Autodesk Inventor part; units mm, degrees
ref_plane "YZ Plane" through (0, 0, 0) normal (1, 0, 0) x (0, 1, 0)
ref_plane "XZ Plane" through (0, 0, 0) normal (0, 1, 0) x (-1, 0, 0)
ref_plane "XY Plane" through (0, 0, 0) normal (0, 0, 1) x (1, 0, 0)
sketch "Sketch1" plane through (0, 0, 0) normal (0, 0, 1) x (1, 0, 0)
  line L0 (0, 0) -> (-228.6, 0)
  line L1 (-228.6, 0) -> (-228.6, 1.5875)
  line L2 (-228.6, 1.5875) -> (-95.25, 25.4)
  line L3 (-95.25, 25.4) -> (0, 25.4)
  line L4 (0, 25.4) -> (0, 0)
  dimension "d0" = 25.4
  dimension "d1" = 228.6
  dimension "d2" = 1.5875
  dimension "d3" = 95.25
extrude "Extrusion1" add sketch "Sketch1" along normal blind 25.4
shell "Shell1" thickness 1.5875 removed faces 2 at (-184.15, 9.525, 8.4667) at (0, 16.9333, 8.4667)
sketch "Sketch2" plane through (0, 0, 0) normal (0, 0, -1) x (-1, 0, 0)
  line L0 (95.25, 25.4) -> (0, 25.4)
  line L1 (0, 25.4) -> (0, 0)
  line L2 (50.8, 25.4) -> (76.2, 25.4)
  line L3 (76.2, 25.4) -> (76.2, 12.7)
  line L4 (76.2, 12.7) -> (50.8, 12.7)
  line L5 (50.8, 12.7) -> (50.8, 25.4)
  dimension "d7" = 25.4
  dimension "d8" = 12.7
  dimension "d9" = 50.8
extrude "Extrusion2" cut sketch "Sketch2" against normal through all
properties part number "Shovel_BottomFrame" material "Aluminum-6061"
CAD build for the part. Positions are in the model's coordinates, mm. A direction names the side the tool comes from. Round coordinates to 2 decimals unless told otherwise and drop trailing zeros. Write each loop counter-clockwise with the first axis right and the second up, starting at its lowest first coordinate (ties: lowest second). Pieces come first, ordered by that corner, then holes. Notation, with made-up numbers: (67.5, 54) -> (82.5, 54) arc R15 cw to (82.5, 80) -> close; hole circle Ø9 at (-25.5, 70). An arc over 180 degrees is marked (long way). Answer as a JSON object with one key per item and string values.
(1) Band-saw the part on B-B, the plane z = 3.5. List the corners of the cut face in (x, y), then the cut area to 3 significant figures.
Reported:
{"outline": "(-228.6, 0) -> (0, 0) -> (0, 1.59) -> (-227.01, 1.59) -> (-227.01, 1.87) -> (-228.6, 1.59) -> close; (-104.14, 23.81) -> (-76.2, 23.81) -> (-76.2, 25.4) -> (-95.25, 25.4) -> close; (-50.8, 23.81) -> (0, 23.81) -> (0, 25.4) -> (-50.8, 25.4) -> close", "area": "481 mm^2"}
(2) Band-saw the part on C-C, the plane x = -32. List the corners of the cut face in (y, z), then the cut area to 3 significant figures.
Reported:
{"outline": "(0, 0) -> (25.4, 0) -> (25.4, 25.4) -> (0, 25.4) -> close; hole (1.59, 1.59) -> (23.81, 1.59) -> (23.81, 23.81) -> (1.59, 23.81) -> close", "area": "151 mm^2"}
(3) Pin check, flat tips, straight feed: P1, Ø6, axis at x = -54, z = 19, coming from the +Y side; P2, Ø1.3, axis at x = -61, z = 24, coming from the +Y side. Stop position of each tip, or through.
Reported:
{"P1": "stops at y = 1.59", "P2": "stops at y = 12.7"}
(4) Probe probe 1 along Z at (x, y) = (-209.5, 4.5); probe 2 along Y at (x, z) = (-201.5, 13.25). List the from-to ranges inside material, lowest first. Write a range as [from, to].
Reported:
{"probe 1": "z = [0, 1.59], [23.81, 25.4]", "probe 2": "y = [0, 1.59]"}
(5) Band-saw the part on D-D, the plane y = 7.5. List the corners of the cut face in (x, z), then the cut area to 3 significant figures.
Reported:
{"outline": "(-195.49, 0) -> (0, 0) -> (0, 1.59) -> (-195.49, 1.59) -> close; (-195.49, 23.81) -> (0, 23.81) -> (0, 25.4) -> (-195.49, 25.4) -> close", "area": "621 mm^2"}
(6) Band-saw the part on A-A, the plane y = 17.75. List the corners of the cut face in (x, z).
Reported:
{"outline": "(-138.09, 0) -> (-76.2, 0) -> (-76.2, 1.59) -> (-138.09, 1.59) -> close; (-138.09, 23.81) -> (-76.2, 23.81) -> (-76.2, 25.4) -> (-138.09, 25.4) -> close; (-50.8, 0) -> (0, 0) -> (0, 1.59) -> (-50.8, 1.59) -> close; (-50.8, 23.81) -> (0, 23.81) -> (0, 25.4) -> (-50.8, 25.4) -> close"}
(7) Two-plate mould, pull along X, no slides. Class faces 1 (the face through (-50.8, 24, 12)), 2 (the face through (-142.481, 16.966, 24.87)), 3 (the face through (-91, 10, 25.4)), 4 (the face through (-76.2, 24, 13)): +X half, -X half, draft (parallel to the pull), parting line (faces both ways), or undercut.
Reported:
{"face 1": "undercut", "face 2": "-X half", "face 3": "draft", "face 4": "undercut"}
(8) Which spindle directions (+Z, -Z, +X, -X, +Y, -Y) get a long thin tool onto all of the face, cutting with end or side? Do faces 5 (the face through (-26, 25.4, 13)), 6 (the face through (-112, 1.588, 13)), 7 (the face through (-90, 23.812, 13)). Say none if no direction does.
Reported:
{"face 5": "+Z, -Z, +X, -X, +Y", "face 6": "+X", "face 7": "+X, -X"}
